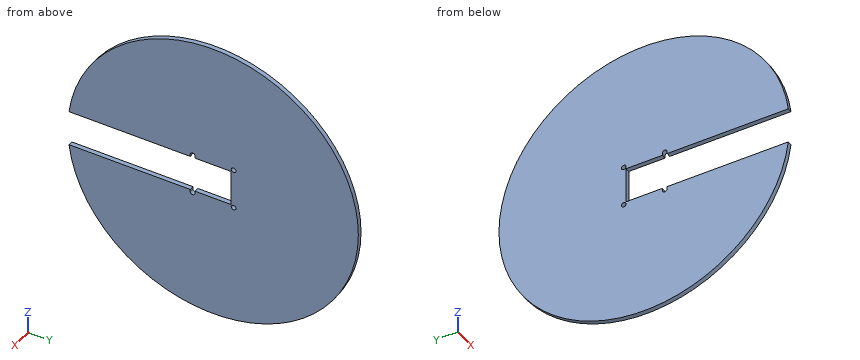
```python
from build123d import *

# Parameters (mm, degrees)
SKETCH1_R           = 1.651
BOSS_EXTRUDE1_DEPTH = 3.175


with BuildPart() as part:
    # Sketch1 → Boss-Extrude1 (new body)
    with BuildSketch(Plane(origin=(0, 0, 0), x_dir=(0, 0, -1), z_dir=(1, 0, 0))):
        with BuildLine():
            Line((-12.7, -12.693314325), (-12.7, 12.7))
            Line((-12.7, 12.7), (12.7, 12.7))
            Line((12.7, 12.7), (12.7, -12.693314325))
            Line((12.7, -12.693314325), (14.351, -12.693314325))
            ThreePointArc((14.351, -12.693314325), (16.008685675, -14.351), (14.351, -16.008685675))
            Line((14.351, -16.008685675), (12.7, -16.008685675))
            Line((12.7, -16.008685675), (12.7, -100.803124952))
            ThreePointArc((12.7, -100.803124952), (0, 101.6), (-12.7, -100.803124952))
            Line((-12.7, -100.803124952), (-12.7, -16.008685675))
            Line((-12.7, -16.008685675), (-14.351, -16.008685675))
            ThreePointArc((-14.351, -16.008685675), (-16.008685675, -14.351), (-14.351, -12.693314325))
            Line((-14.351, -12.693314325), (-12.7, -12.693314325))
        make_face()
        with Locations((-14.351, 14.351)):
            Circle(SKETCH1_R, mode=Mode.SUBTRACT)
        with Locations((14.351, 14.351)):
            Circle(SKETCH1_R, mode=Mode.SUBTRACT)
    extrude(amount=BOSS_EXTRUDE1_DEPTH)


solid = part.part
```
Can you work these out from the model? Positions are in its coordinate system, mm. Give positions to 0.01 mm unless a question says otherwise; leave off trailing zeros. Order: outer loops, then holes, each group sorted by start corner. A loop starts at its lowest first (then second) coordinate and runs counter-clockwise, first axis right, second up. Notation, with made-up numbers: M 89,63.25 L 122,63.25 A20 cw 122,72.25 Z; hole C 12,62.25 d9. An arc over 180 degrees is marked long. Write item = value, one per line. Start each with the question number.
Q1. Suppose I cut it at B-B (x = 1.8). Write out the boundary of the cut face in (y, z), plus the area to 3 significant figures.
Q2. Suppose I cut it at D-D (y = 59.5). Write out the boundary of the cut face in (x, z) (3 decimals), plus the area to 3 significant figures.
Q3. Suppose I cut it at A-A (y = 0). Write out the boundary of the cut face in (x, z) (3 decimals), plus the area to 3 significant figures.
Q4. I need wall thicknesses on probe 1 along Z at (x, y) = (1.2, -1.5); probe 2 along Y at (x, z) = (2.1, -14.5); probe 3 along Z at (x, y) = (0.6, -89.5). Which ranges of each line are inside material? Lowest first, please. Write a range as [from, to].
Q5. Will these pins go through, and if not, where does the flat tip stop? pin 1 Ø1.6 at (x, y) = (2, -65) entering from -Z; pin 2 Ø1.3 at (x, z) = (2.5, -13.5) entering from +Y; pin 3 Ø1 at (x, y) = (1.5, -0.5) entering from -Z; pin 4 Ø3 at (y, z) = (14.351, 14.351) entering from +X.
Q6. Suppose I cut it at C-C (z = 0). Write out the boundary of the cut face in (x, y) (3 decimals), plus the area to 3 significant figures.
Check result:
q1.outline = M -100.8,-12.7 A101.6 ccw long -100.8,12.7 L -16.01,12.7 L -16.01,14.35 A1.66 cw -12.69,14.35 L -12.69,12.7 L 12.7,12.7 L 12.7,-12.7 L -12.69,-12.7 L -12.69,-14.35 A1.66 cw -16.01,-14.35 L -16.01,-12.7 Z; hole C 14.35,-14.35 d3.3; hole C 14.35,14.35 d3.3
q1.area = 29,500 mm2
q2.outline = M 0,-82.355 L 3.175,-82.355 L 3.175,82.355 L 0,82.355 Z
q2.area = 523 mm2
q3.outline = M 0,-101.6 L 3.175,-101.6 L 3.175,-12.7 L 0,-12.7 Z; M 0,12.7 L 3.175,12.7 L 3.175,101.6 L 0,101.6 Z
q3.area = 565 mm2
q4.probe_1 = [-101.59, -12.7], [12.7, 101.59]
q4.probe_2 = [-100.56, -16], [-12.7, 12.71], [16, 100.56]
q4.probe_3 = [-48.09, -12.7], [12.7, 48.09]
q5.pin_1 = -78.75
q5.pin_2 = 100.78
q5.pin_3 = -101.6
q5.pin_4 = through
q6.outline = M 0,12.7 L 3.175,12.7 L 3.175,101.6 L 0,101.6 Z
q6.area = 282 mm2
